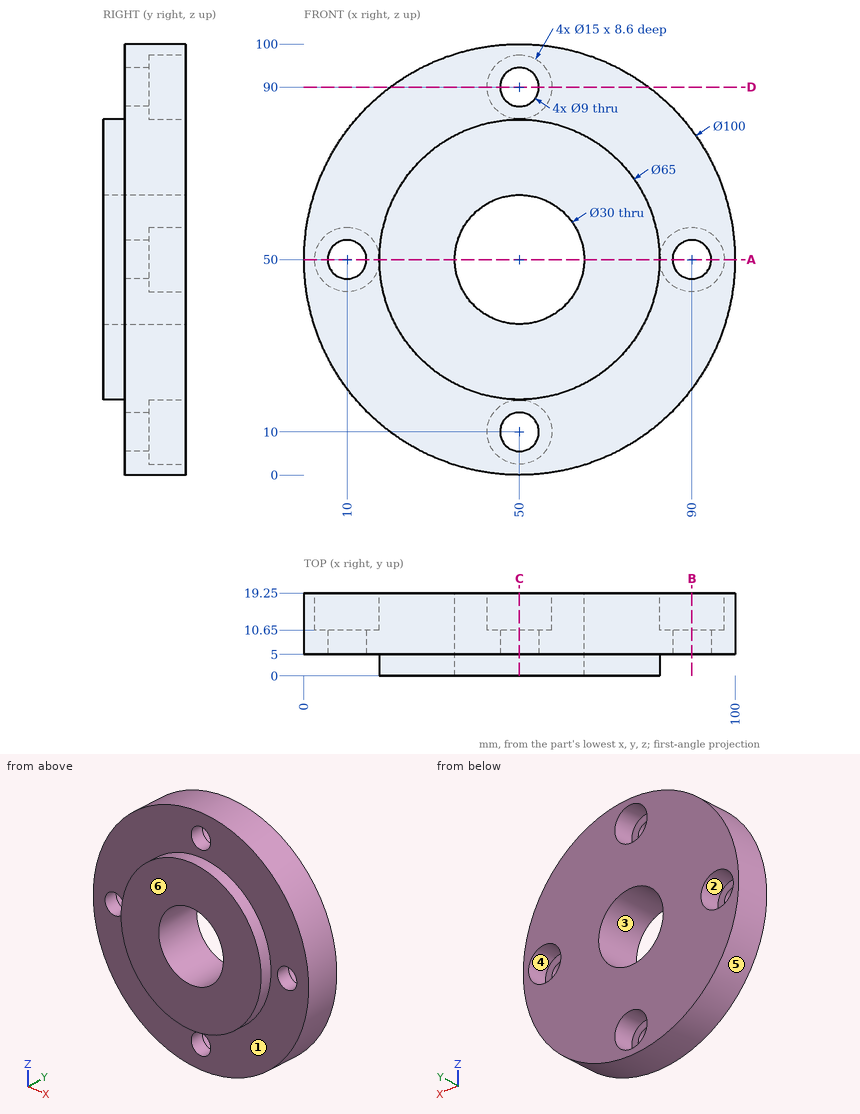
Source: three-view drawing plus pictorial views. Frame: mm from the lowest corner of the part. A direction names the side the tool comes from. Round coordinates to 2 decimals unless told otherwise and drop trailing zeros. Loops run counter-clockwise (first coordinate to the right, second up) from the corner with the lowest first, then second, coordinate; pieces in that order, holes last.
Item 1: Mould query, pull axis Z, two halves, no side actions, for the marked faces 4, 5 and 6. Classes: released by +Z, released by -Z, zero draft, split by the parting line, or undercut.
Checked values:
face 4: undercut
face 5: split by the parting line
face 6: zero draft
Item 2: Line query: L1, parallel to X at y = 7.7, z = 50; L2, parallel to X at y = 14, z = 50; L3, parallel to X at y = 4.25, z = 50. Output: solid intervals per line, ascending.
Checked values:
L1: x = 0 to 5.5, 14.5 to 35, 65 to 85.5, 94.5 to 100
L2: x = 0 to 2.5, 17.5 to 35, 65 to 82.5, 97.5 to 100
L3: x = 17.5 to 35, 65 to 82.5
Item 3: Section A-A, the plane z = 50. Output: boundary loops of the cut face in (x, y), plus the area to 3 significant figures.
Checked values:
outline: (0, 5) - (5.5, 5) - (5.5, 10.65) - (2.5, 10.65) - (2.5, 19.25) - (0, 19.25) - close; (14.5, 5) - (17.5, 5) - (17.5, 0) - (35, 0) - (35, 19.25) - (17.5, 19.25) - (17.5, 10.65) - (14.5, 10.65) - close; (65, 0) - (82.5, 0) - (82.5, 5) - (85.5, 5) - (85.5, 10.65) - (82.5, 10.65) - (82.5, 19.25) - (65, 19.25) - close; (94.5, 5) - (100, 5) - (100, 19.25) - (97.5, 19.25) - (97.5, 10.65) - (94.5, 10.65) - close
area: 813 mm2
Item 4: Section B-B, the plane x = 90. Output: boundary loops of the cut face in (y, z), plus the area to 3 significant figures.
Checked values:
outline: (5, 20) - (19.25, 20) - (19.25, 42.5) - (10.65, 42.5) - (10.65, 45.5) - (5, 45.5) - close; (5, 54.5) - (10.65, 54.5) - (10.65, 57.5) - (19.25, 57.5) - (19.25, 80) - (5, 80) - close
area: 675 mm2
Item 5: Contact query for flat-ended pins moving along their axis: P1, Ø7.5, axis at x = 90.5, z = 52, coming from the +Y side; P2, Ø12, axis at x = 52, z = 89.5, coming from the +Y side; P3, Ø1.5, axis at x = 62.5, y = 4.5, coming from the -Z side; P4, Ø6, axis at y = 14.5, z = 62.5, coming from the -X side. Output: stop coordinate, or through.
Checked values:
P1: stops at y = 10.65
P2: stops at y = 19.25
P3: stops at z = 1.45
P4: stops at x = 0.91
Item 6: Section D-D, the plane z = 90. Output: boundary loops of the cut face in (x, y), plus the area to 3 significant figures.
Checked values:
outline: (20, 5) - (45.5, 5) - (45.5, 10.65) - (42.5, 10.65) - (42.5, 19.25) - (20, 19.25) - close; (54.5, 5) - (80, 5) - (80, 19.25) - (57.5, 19.25) - (57.5, 10.65) - (54.5, 10.65) - close
area: 675 mm2
Item 7: Section C-C, the plane x = 50. Output: boundary loops of the cut face in (y, z).
Checked values:
outline: (0, 17.5) - (5, 17.5) - (5, 14.5) - (10.65, 14.5) - (10.65, 17.5) - (19.25, 17.5) - (19.25, 35) - (0, 35) - close; (0, 65) - (19.25, 65) - (19.25, 82.5) - (10.65, 82.5) - (10.65, 85.5) - (5, 85.5) - (5, 82.5) - (0, 82.5) - close; (5, 0) - (19.25, 0) - (19.25, 2.5) - (10.65, 2.5) - (10.65, 5.5) - (5, 5.5) - close; (5, 94.5) - (10.65, 94.5) - (10.65, 97.5) - (19.25, 97.5) - (19.25, 100) - (5, 100) - close
Item 8: Reachability of the marked faces 1, 2 and 3 from +Z, -Z, +X, -X, +Y, -Y: full face, straight path, thin tool, end or side. Return the list, or none.
Checked values:
face 1: -Y
face 2: +Y
face 3: +Y, -Y
